The listing builds one solid part. Answer for the finished solid, in the listing's coordinates (mm). Give positions to 0.01 mm unless a question says otherwise; leave off trailing zeros. Loops run counter-clockwise (first coordinate to the right, second up) from the corner with the lowest first, then second, coordinate; pieces in that order, holes last. Notation, with made-up numbers: M -39.5,-34.75 L -4.5,-34.75 A19 cw -4.5,-9.75 Z; hole C 28.5,88.5 d7. An arc over 180 degrees is marked long. One line per item, written item: value. Start each with the question number.
Q1. The mould has two halves that part along Y. Classify faces 1 (the flat face through (0, 2, 6)), 2 (the flat face through (-1, 2, 0)), 3 (the flat face through (1, -150, 4)): +Y half, -Y half, draft (parallel to the pull), parting line (faces both ways), or undercut.
Q2. A cutting plane is placed at A-A, the plane x = 22. Determine the outline of the cut face in (y, z), and give its area (3 significant figures).
Q3. A cutting plane is placed at B-B, the plane y = 3. Determine the outline of the cut face in (x, z).
Q4. Consider L1, parallel to X at y = -16, z = 7.5; L2, parallel to Y at x = -18.5, z = 6.25; L3, parallel to Z at x = -22, y = 109. Determine where each line is inside the solid, lowest interval first.
Autodesk Inventor part; units mm, degrees
ref_plane "YZ Plane" through (0, 0, 0) normal (1, 0, 0) x (0, 1, 0)
ref_plane "XZ Plane" through (0, 0, 0) normal (0, 1, 0) x (-1, 0, 0)
ref_plane "XY Plane" through (0, 0, 0) normal (0, 0, 1) x (1, 0, 0)
sketch "Sketch1" plane through (0, 0, 0) normal (0, 0, 1) x (1, 0, 0)
  line L0 (-37.5, 150) -> (37.5, 150)
  line L1 (37.5, 150) -> (37.5, -150)
  line L2 (37.5, -150) -> (-37.5, -150)
  line L3 (-37.5, -150) -> (-37.5, 150)
  point P0 (0, 0)
  dimension "d0" = 75
  dimension "d1" = 300
  dimension "d2" = 150
  dimension "d3" = 37.5
extrude "Extrusion1" add sketch "Sketch1" along normal blind 8
sketch "Sketch2" plane through (0, 0, 8) normal (0, 0, 1) x (1, 0, 0)
  line L0 (-28.5, 143.5) -> (28.5, 143.5)
  line L1 (28.5, 143.5) -> (28.5, -143.5)
  line L2 (28.5, -143.5) -> (-28.5, -143.5)
  line L3 (-28.5, -143.5) -> (-28.5, 143.5)
  point P0 (0, 0)
  dimension "d6" = 57
  dimension "d7" = 287
  dimension "d8" = 143.5
  dimension "d9" = 28.5
extrude "Extrusion2" cut sketch "Sketch2" against normal blind 2
properties part number "filter top plate" material "Aluminum 6061-AHC"
Answer block:
1. face 1: undercut
1. face 2: draft
1. face 3: -Y half
2. outline: M -150,0 L 150,0 L 150,8 L 143.5,8 L 143.5,6 L -143.5,6 L -143.5,8 L -150,8 Z
2. area: 1,830 mm^2
3. outline: M -37.5,0 L 37.5,0 L 37.5,8 L 28.5,8 L 28.5,6 L -28.5,6 L -28.5,8 L -37.5,8 Z
4. L1: -37.5 to -28.5, 28.5 to 37.5
4. L2: -150 to -143.5, 143.5 to 150
4. L3: 0 to 6
